The model under review builds one solid part; all positions refer to its coordinate system, in mm. Face numbers are marked on the shaded views. A direction names the side the tool comes from. Coordinates: 2 decimals unless noted, no trailing zeros. Loops run counter-clockwise (first coordinate to the right, second up) from the corner with the lowest first, then second, coordinate; pieces in that order, holes last. Notation, with made-up numbers: M 50.5,33.25 L 65.5,33.25 A13 cw 65.5,49.25 Z; hole C -6.75,33 d7. An arc over 180 degrees is marked long. One line per item, written item: value.
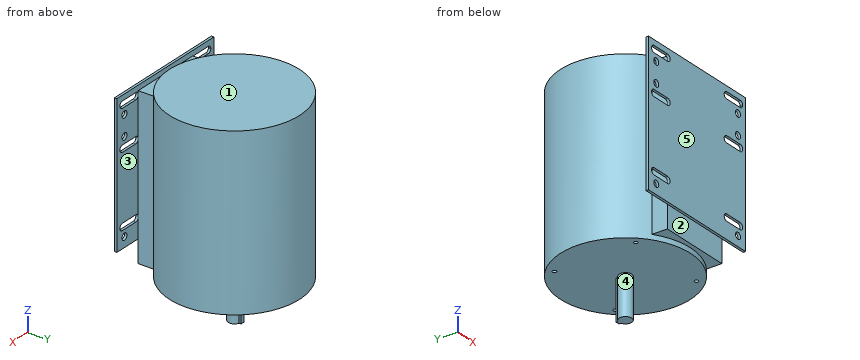
Autodesk Inventor part; units mm, degrees
ref_plane "YZ Plane" through (0, 0, 0) normal (1, 0, 0) x (0, 1, 0)
ref_plane "XZ Plane" through (0, 0, 0) normal (0, 1, 0) x (-1, 0, 0)
ref_plane "XY Plane" through (0, 0, 0) normal (0, 0, 1) x (1, 0, 0)
sketch "Sketch1" plane through (0, 0, 0) normal (0, 0, 1) x (1, 0, 0)
  circle A0 centre (0, 0) radius 7.9375
  line L0 (-2.4257, 7.5578) -> (-2.4257, 10.0978)
  line L1 (-2.4257, 10.0978) -> (2.4257, 10.0978)
  line L2 (2.4257, 10.0978) -> (2.4257, 7.5578)
  point P0 (0, 10.0978)
  dimension "d0" = 15.875
  dimension "d1" = 2.54
  dimension "d2" = 4.8514
extrude "Extrusion1" add sketch "Sketch1" along normal blind 50.8
sketch "Sketch2" plane through (0, 0, 50.8) normal (0, 0, 1) x (1, 0, 0)
  circle A0 centre (0, 0) radius 82.55
  dimension "d5" = 165.1
extrude "Extrusion2" add sketch "Sketch2" along normal blind 212.7758
sketch "Sketch3" plane through (0, 0, 50.8) normal (0, 0, -1) x (-1, 0, 0)
  circle A0 centre (0, 0) radius 73.025
  arc A1 (-2.4257, 7.5578) -> (2.4257, 7.5578) centre (0, 0) ccw
  line L0 (0, 0) -> (51.6365, 51.6365)
  line L1 (0, 0) -> (73.025, 0) construction
  line L2 (0, 0) -> (51.6365, -51.6365)
  line L3 (0, 0) -> (73.025, 0) construction
  line L4 (0, 0) -> (-51.6365, 51.6365)
  line L5 (0, 0) -> (73.025, 0) construction
  line L6 (0, 0) -> (-51.6365, -51.6365)
  line L7 (0, 0) -> (73.025, 0) construction
  dimension "d8" = 146.05
  dimension "d9" = 45
  dimension "d10" = 45
  dimension "d11" = 135
  dimension "d12" = 135
hole "Hole1" at (51.6365, 51.6365, 50.8) at (-51.6365, 51.6365, 50.8) at (-51.6365, -51.6365, 50.8) at (51.6365, -51.6365, 50.8) direction (0, 0, 1) diameter 4.9784 depth 19.05 tip angle 118
ref_plane "Work Plane2" through (0, -82.55, 50.8) normal (0, 1, 0) x (-1, 0, 0)
sketch "Sketch4" plane through (0, -82.55, 50.8) normal (0, 1, 0) x (-1, 0, 0)
  line L0 (82.55, 212.7758) -> (-82.55, 212.7758)
  line L1 (-82.55, 0) -> (82.55, 0)
  line L2 (82.55, 0) -> (82.55, 177.8)
  line L3 (-82.55, 0) -> (-82.55, 177.8)
  line L4 (-46.355, 6.35) -> (46.355, 6.35)
  line L5 (46.355, 6.35) -> (46.355, 206.4258)
  line L6 (46.355, 206.4258) -> (-46.355, 206.4258)
  line L7 (-46.355, 206.4258) -> (-46.355, 6.35)
  point P0 (0, -50.8)
  point P1 (0, 6.35)
  dimension "d20" = 200.0758
  dimension "d21" = 6.35
  dimension "d22" = 92.71
extrude "Extrusion3" add sketch "Sketch4" along normal blind 25.4 and the other way blind 5.2324
ref_plane "Work Plane7" through (0, -90.9574, 50.8) normal (0, -1, 0) x (1, 0, 0)
sketch "Sketch5" plane through (0, -90.9574, 50.8) normal (0, -1, 0) x (1, 0, 0)
  line L0 (82.55, 212.7758) -> (-82.55, 212.7758)
  line L1 (82.55, 212.7758) -> (-82.55, 212.7758)
  line L2 (-82.55, 212.7758) -> (-82.55, 34.9758)
  line L3 (-82.55, 34.9758) -> (82.55, 34.9758)
  line L4 (82.55, 34.9758) -> (82.55, 212.7758)
  point P0 (0, -50.8)
  dimension "d54" = 177.8
  dimension "d55" = 165.1
extrude "Extrusion4" add sketch "Sketch5" against normal blind 3.175
ref_plane "Work Plane9" through (0, -94.1324, 50.8) normal (0, -1, 0) x (1, 0, 0)
sketch "Sketch6" plane through (0, -94.1324, 50.8) normal (0, -1, 0) x (1, 0, 0)
  circle A0 centre (69.5575, 189.0141) radius 4.2291
  line L0 (73.2282, 206.0194) -> (50.3174, 206.0194)
  line L1 (50.3174, 197.5612) -> (73.2282, 197.5612)
  line L2 (77.4117, 201.1711) -> (77.4117, 202.4095)
  arc A1 (73.2282, 197.5612) -> (73.2282, 206.0194) centre (73.2282, 201.7903) ccw
  arc A2 (50.3174, 206.0194) -> (50.3174, 197.5612) centre (50.3174, 201.7903) ccw
  circle A3 centre (69.5575, 163.6903) radius 4.2291
  line L3 (73.2405, 146.685) -> (50.3297, 146.685)
  line L4 (50.3297, 155.1432) -> (73.2405, 155.1432)
  arc A4 (73.2405, 146.685) -> (73.2405, 155.1432) centre (73.2405, 150.9141) ccw
  arc A5 (50.3297, 155.1432) -> (50.3297, 146.685) centre (50.3174, 150.9141) ccw
  arc A6 (73.2405, 56.1594) -> (73.2405, 64.6176) centre (73.2405, 60.3885) ccw
  line L5 (50.3297, 56.1594) -> (73.2405, 56.1594)
  line L6 (73.2405, 64.6176) -> (50.3297, 64.6176)
  arc A7 (50.3297, 64.6176) -> (50.3297, 56.1594) centre (50.3174, 60.3885) ccw
  circle A8 centre (69.5575, 47.6123) radius 4.2291
  circle A9 centre (-69.3613, 189.0141) radius 4.2291
  line L7 (-73.0443, 206.0194) -> (-50.1335, 206.0194)
  line L8 (-50.1335, 197.5612) -> (-73.0443, 197.5612)
  line L9 (-77.2278, 201.1711) -> (-77.2278, 202.4095)
  arc A10 (-73.0443, 206.0194) -> (-73.0443, 197.5612) centre (-73.0443, 201.7903) ccw
  arc A11 (-50.1335, 197.5612) -> (-50.1335, 206.0194) centre (-50.1335, 201.7903) ccw
  arc A12 (-73.0443, 155.1432) -> (-73.0443, 146.685) centre (-73.0443, 150.9141) ccw
  line L10 (-50.1335, 155.1432) -> (-73.0443, 155.1432)
  line L11 (-73.0443, 146.685) -> (-50.1335, 146.685)
  arc A13 (-50.1335, 146.685) -> (-50.1335, 155.1432) centre (-50.1335, 150.9141) ccw
  circle A14 centre (-69.3613, 163.6903) radius 4.2291
  circle A15 centre (-69.3613, 47.6123) radius 4.2291
  line L12 (-50.1335, 56.1594) -> (-73.0443, 56.1594)
  line L13 (-73.0443, 64.6176) -> (-50.1335, 64.6176)
  arc A16 (-73.0443, 64.6176) -> (-73.0443, 56.1594) centre (-73.0443, 60.3885) ccw
  arc A17 (-50.1335, 56.1594) -> (-50.1335, 64.6176) centre (-50.1335, 60.3885) ccw
  line L14 (-82.55, 212.7758) -> (-82.55, 34.9758)
  line L15 (82.55, 212.7758) -> (-82.55, 212.7758)
  line L16 (82.55, 34.9758) -> (82.55, 212.7758)
  line L17 (82.55, 212.7758) -> (82.55, 34.9758)
  point P0 (0, -50.8)
  point P1 (-61.5889, 206.0194)
  point P2 (61.7728, 206.0194)
  point P3 (-61.5889, 197.5612)
  point P4 (61.7728, 197.5612)
  point P5 (-61.5889, 155.1432)
  point P6 (61.7851, 155.1432)
  dimension "d31" = 8.4582
  dimension "d38" = 8.4582
  dimension "d39" = 8.4582
  dimension "d40" = 22.9108
  dimension "d41" = 8.4582
  dimension "d51" = 8.5471
  dimension "d56" = 50.8762
  dimension "d57" = 12.7762
  dimension "d58" = 6.7564
  dimension "d59" = 12.7762
  dimension "d60" = 90.5256
  dimension "d62" = 9.3218
extrude "Extrusion5" cut sketch "Sketch6" against normal blind 6.35 contours A0 | A1 L2 L1 A2 L0 | A3 | L3 A5 L4 A4 | L5 A7 L6 A6 | A8 | A9 | L7 A11 L8 A10 L9 | L10 A13 L11 A12 | A14 | A15 | L12 A16 L13 A17
sketch "Sketch7" plane through (0, -87.7824, 50.8) normal (0, -1, 0) x (1, 0, 0)
  point P0 (0, -50.8)
equation "\"d3\" = ShaftL"
equation "\"d5\" = MotoD"
equation "\"d6\" = MotoL"
equation "\"ShaftL\" = 50.8"
equation "\"MotoD\" = 165.1"
equation "\"MotoL\" = 212.7758"
properties part number "Motor4"
(1) Add section A-A on y = 0. State the section outline as (x, z) points.
Checks:
outline: M -82.55,50.8 L -7.94,50.8 L -7.94,0 L 7.94,0 L 7.94,50.8 L 82.55,50.8 L 82.55,263.58 L -82.55,263.58 Z
(2) Add section D-D on x = 23. State the section outline as (y, z) points, then the cut area to 3 significant figures.
Checks:
outline: M -90.96,85.78 L -87.78,85.78 L -87.78,57.15 L -79.28,57.15 L -79.28,50.8 L 79.28,50.8 L 79.28,263.58 L -79.28,263.58 L -79.28,257.23 L -87.78,257.23 L -87.78,263.58 L -90.96,263.58 Z
area: 36,000 mm^2
(3) Insertion check: pin 1 Ø1.3 at (y, z) = (9, 31) entering from -X; pin 2 Ø6 at (y, z) = (5, 76) entering from -X; pin 3 Ø2.5 at (x, z) = (-1, 30) entering from +Y; pin 4 Ø2 at (y, z) = (22.5, 48.5) entering from -X. Each pin has a flat end and moves straight along its axis. Give the tip position at first contact, or say it passes through.
Checks:
pin 1: x = -2.43
pin 2: x = -82.53
pin 3: y = 10.1
pin 4: through
(4) To check wall thickness, follow L1, parallel to Z at x = 24, y = -79.5; L2, parallel to Y at x = 38, z = 182.5; L3, parallel to Y at x = 68, z = 228. State the ranges of each line that lie inside material, in increasing order. Write a range as [from, to].
Checks:
L1: [57.15, 257.23]
L2: [-90.96, 73.28]
L3: [-90.96, -87.78], [-46.8, 46.8]
(5) Add section B-B on z = 136. State the section outline as (x, y) points (3 decimals).
Checks:
outline: M -82.55,-90.957 L 82.55,-90.957 L 82.55,-87.782 L 46.355,-87.782 L 46.355,-68.306 A82.55 ccw long -46.355,-68.306 L -46.355,-87.782 L -82.55,-87.782 Z
(6) Add section C-C on x = -30.5. State the section outline as (y, z) points.
Checks:
outline: M -90.96,85.78 L -87.78,85.78 L -87.78,57.15 L -76.71,57.15 L -76.71,50.8 L 76.71,50.8 L 76.71,263.58 L -76.71,263.58 L -76.71,257.23 L -87.78,257.23 L -87.78,263.58 L -90.96,263.58 Z
(7) Draft analysis for pull direction Y (two halves, no side actions). For the marked faces 3, 4 and 5, state which applies: pulls with the +Y half, pulls with the -Y half, needs draft (parallel to the pull), parting line crosses it, or undercut.
Checks:
face 3: undercut
face 4: parting line crosses it
face 5: pulls with the -Y half
(8) Tool access review of the marked faces 1 and 2: name each direction out of +Z, -Z, +X, -X, +Y, -Y from which nothing blocks a thin tool from reaching the whole face with its end or side.
Checks:
face 1: +Z, +X, -X, +Y, -Y
face 2: -Z, +X, -X, -Y
